Input: part model. Units: mm. Frame: model coordinates. A direction names the side the tool comes from. Round coordinates to 2 decimals unless told otherwise and drop trailing zeros. Loops run counter-clockwise (first coordinate to the right, second up) from the corner with the lowest first, then second, coordinate; pieces in that order, holes last. Notation, with made-up numbers: M -22,74.5 L 30,74.5 A30 cw 30,106.5 Z; hole C 43,27 d10. An arc over 180 degrees is marked long. Return JSON: item names as keys, results as strings. Group by question number.
1) Section A-A (x = 0). Output: boundary loops of the cut face in (y, z).
2) Contact query for flat-ended pins moving along their axis: P1, Ø1.5, axis at x = -5, z = -8, coming from the -Y side; P2, Ø1.5, axis at y = 4, z = -7, coming from the +X side; P3, Ø1, axis at x = -8.5, y = 6, coming from the -Z side. Output: stop coordinate, or through.
3) Material intervals for line 1 (X direction, y = 5.45, z = 0); line 2 (Y direction, x = 5.75, z = -7.25), sorted ascending. Write a range as from..to.
4) Mould query, pull axis X, two halves, no side actions, for faces 3 (the face through (0.6, 6.5, -8.8)), 4 (the face through (12.443, 6.465, 3.918)), 5 (the face through (11, 0, 3)), 6 (the face through (-9, 6, 0)). Classes: +X half, -X half, draft (parallel to the pull), parting line (faces both ways), or undercut.
5) Section C-C (y = 2.25). Output: boundary loops of the cut face in (x, z).
6) Access query for faces 1 (the face through (10.316, 1.972, 7.91)), 2 (the face through (7, 6, 0)). Directions: +Z, -Z, +X, -X, +Y, -Y. A direction counts if a zero-diameter tool reaches every point of the face in a straight line with its end or side. Return the directions, or none.
7) Section D-D (x = -8). Output: boundary loops of the cut face in (y, z).
8) Section B-B (z = -8). Output: boundary loops of the cut face in (x, y), plus the area to 3 significant figures.
Autodesk Inventor part; units mm, degrees
ref_plane "YZ Plane" through (0, 0, 0) normal (1, 0, 0) x (0, 1, 0)
ref_plane "XZ Plane" through (0, 0, 0) normal (0, 1, 0) x (-1, 0, 0)
ref_plane "XY Plane" through (0, 0, 0) normal (0, 0, 1) x (1, 0, 0)
sketch "Sketch1" plane through (0, 0, 0) normal (0, 1, 0) x (-1, 0, 0)
  circle A0 centre (0, 0) radius 11
  circle A1 centre (0, 0) radius 13
  dimension "d0" = 22
  dimension "d1" = 26
extrude "Extrusion1" add sketch "Sketch1" along normal blind 4
sketch "Sketch2" plane through (0, 4, 0) normal (0, 1, 0) x (1, 0, 0)
  circle A0 centre (0, 0) radius 13.0451
extrude "Extrusion2" add sketch "Sketch2" along normal blind 5
sketch "Sketch3" plane through (0, 9, 0) normal (0, 1, 0) x (1, 0, 0)
  circle A0 centre (0, 0) radius 8
  point P0 (-8, 0)
  point P1 (0, 8)
  point P2 (8, 0)
  point P3 (0, -8)
  dimension "d6" = 16
hole "Hole1" at (-8, 9, 0) at (0, 9, -8) at (8, 9, 0) at (0, 9, 8) direction (0, -1, 0) diameter 2 end through all
properties part number "General Mount"
Returned:
{
 "1": {"outline": "M 0,-13 L 4,-13 L 4,-13.05 L 9,-13.05 L 9,-9 L 4,-9 L 4,-11 L 0,-11 Z; M 0,11 L 4,11 L 4,9 L 9,9 L 9,13.05 L 4,13.05 L 4,13 L 0,13 Z; M 4,-7 L 9,-7 L 9,7 L 4,7 Z"},
 "2": {"P1": "stops at y = 4", "P2": "stops at x = 11.45", "P3": "stops at z = -10.3"},
 "3": {"line 1": "x = -13.05..-9, -7..7, 9..13.05", "line 2": "y = 4..9"},
 "4": {"face 3": "undercut", "face 4": "parting line", "face 5": "draft", "face 6": "undercut"},
 "5": {"outline": "C 0,0 d26; hole C 0,0 d22"},
 "6": {"face 1": "-Y", "face 2": "+Y, -Y"},
 "7": {"outline": "M 0,-10.25 L 4,-10.25 L 4,-10.3 L 9,-10.3 L 9,-1 L 4,-1 L 4,-7.55 L 0,-7.55 Z; M 0,7.55 L 4,7.55 L 4,1 L 9,1 L 9,10.3 L 4,10.3 L 4,10.25 L 0,10.25 Z"},
 "8": {"outline": "M -10.3,4 L -10.25,4 L -10.25,0 L -7.55,0 L -7.55,4 L -1,4 L -1,9 L -10.3,9 Z; M 1,4 L 7.55,4 L 7.55,0 L 10.25,0 L 10.25,4 L 10.3,4 L 10.3,9 L 1,9 Z", "area": "115 mm^2"}
}
